Study the drawing (mm; zero at the part's minimum x, y, z) and answer. A direction names the side the tool comes from. Coordinates: 2 decimals unless noted, no trailing zeros. Order: outer loops, then holes, each group sorted by start corner. A loop starts at its lowest first (then second) coordinate and runs counter-clockwise, first axis right, second up. Notation, with made-up numbers: (-32.75, -13) -> (-4.75, -13) arc R19 ccw to (-4.75, 21) -> close; hole circle Ø9 at (82.25, 58.25). An arc over 180 degrees is marked (long way). Write each question's results on one line, items separated by ' | '. Start each with the question number.
(1) The part is cut by section A-A, the plane y = 17.65. Give the vertices of the cut face in (x, z) (3 decimals).
(2) A tool of negligible diameter and unlimited length cuts with its end or side. For the marked faces 4 and 5, from which of +Z, -Z, +X, -X, +Y, -Y can it reach the whole face along a straight path? Write none if from no direction.
(3) The part is cut by section B-B, the plane z = 18.25. Give the vertices of the cut face in (x, y) (3 decimals).
(4) Straight lines are drawn through the part: L1, parallel to X at y = 17.65, z = 16 (3 decimals); L2, parallel to X at y = 18.5, z = 18.25. For each, find the intervals that lie inside material, in ascending order.
(5) The part is cut by section C-C, the plane x = 48. Give the vertices of the cut face in (y, z), then the cut area to 3 significant figures.
(6) Determine the mould class of the marked faces 1, 2 and 3 for opening direction Y: +Y half, -Y half, draft (parallel to the pull), parting line (faces both ways), or undercut.
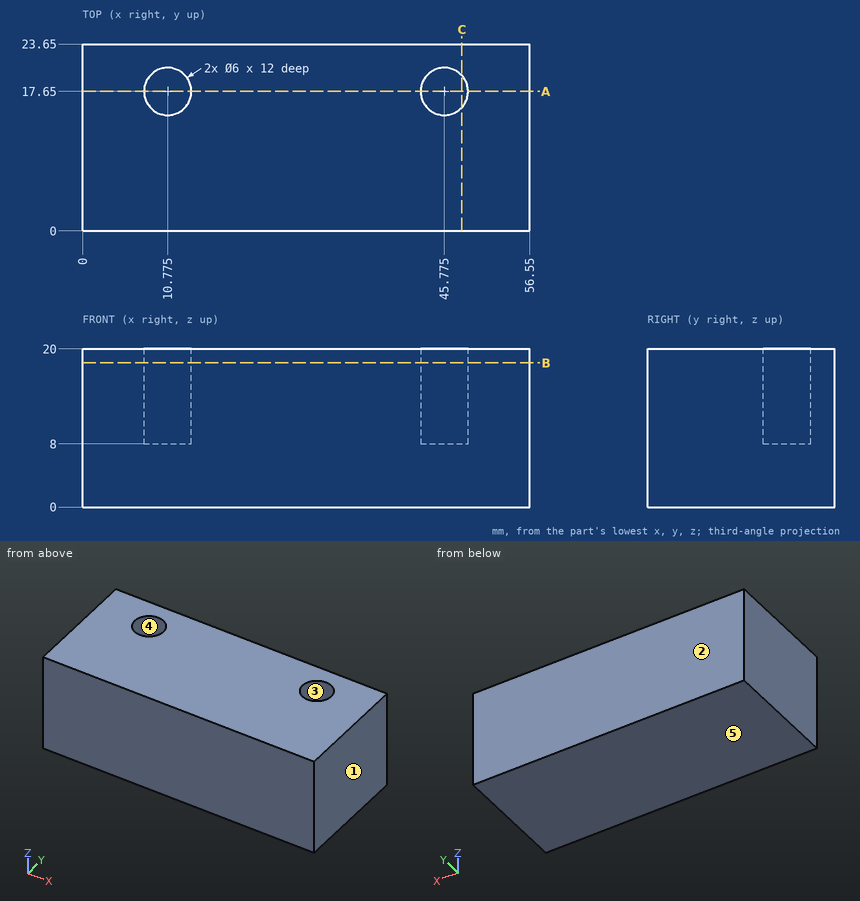
Established:
1) outline: (0, 0) -> (56.55, 0) -> (56.55, 20) -> (48.775, 20) -> (48.775, 8) -> (42.775, 8) -> (42.775, 20) -> (13.775, 20) -> (13.775, 8) -> (7.775, 8) -> (7.775, 20) -> (0, 20) -> close
2) face 4: +Z | face 5: -Z, +X, -X, +Y, -Y
3) outline: (0, 0) -> (56.55, 0) -> (56.55, 23.65) -> (0, 23.65) -> close; hole circle Ø6 at (10.775, 17.65); hole circle Ø6 at (45.775, 17.65)
4) L1: x = 0 to 7.775, 13.775 to 42.775, 48.775 to 56.55 | L2: x = 0 to 7.9, 13.65 to 42.9, 48.65 to 56.55
5) outline: (0, 0) -> (23.65, 0) -> (23.65, 20) -> (19.66, 20) -> (19.66, 8) -> (15.64, 8) -> (15.64, 20) -> (0, 20) -> close | area: 425 mm^2
6) face 1: draft | face 2: +Y half | face 3: undercut
